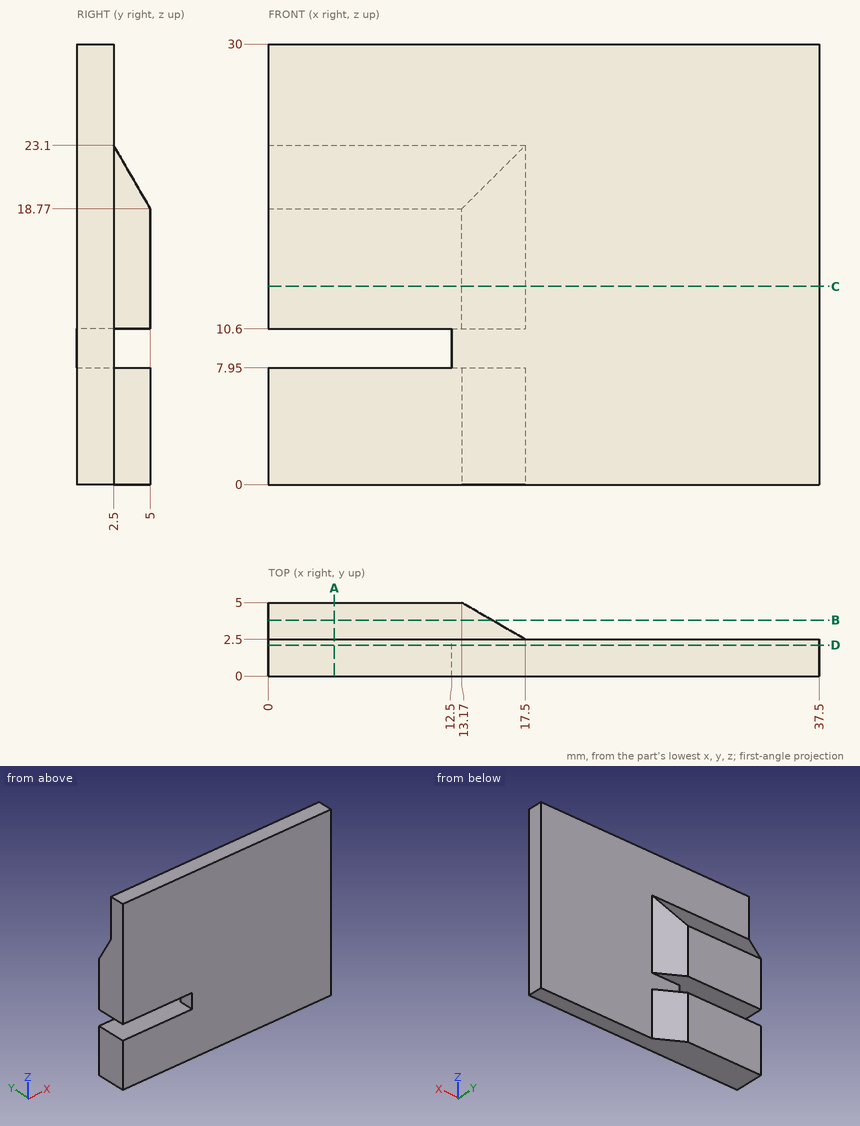
Here's the drawing with two shaded views (mm, measured from the low corner). I have some questions. Coordinates: 2 decimals unless noted, no trailing zeros. Write each loop counter-clockwise with the first axis right and the second up, starting at its lowest first coordinate (ties: lowest second). Pieces come first, ordered by that corner, then holes. Notation, with made-up numbers: M 38.5,-20.75 L 68.5,-20.75 A19 cw 68.5,13.25 Z; hole C 51,65 d4. An arc over 180 degrees is marked long. Use one line per item in the form item = value.
Q1. I need wall thicknesses on line 1 along Z through (x, y) = (4.5, 0.5); line 2 along Y through (x, z) = (23.5, 6.5); line 3 along X through (y, z) = (3.45, 16.75) (1 decimal). Which ranges of each line are inside material? Lowest first, please. Write a range as from..to.
Model answer:
line_1 = 0..7.95, 10.6..30
line_2 = 0..2.5
line_3 = 0..15.9
Q2. If we section it at A-A (x = 4.5): Write out the boundary of the cut face in (y, z).
Model answer:
outline = M 0,0 L 5,0 L 5,7.95 L 0,7.95 Z; M 0,10.6 L 5,10.6 L 5,18.77 L 2.5,23.1 L 2.5,30 L 0,30 Z
Q3. If we section it at B-B (y = 3.8): Write out the boundary of the cut face in (x, z), then the cut area to 4 significant figures.
Model answer:
outline = M 0,0 L 15.25,0 L 15.25,7.95 L 0,7.95 Z; M 0,10.6 L 15.25,10.6 L 15.25,20.85 L 0,20.85 Z
area = 277.5 mm^2
Q4. If we section it at D-D (y = 2.1): Write out the boundary of the cut face in (x, z), then the cut area to 3 significant figures.
Model answer:
outline = M 0,0 L 37.5,0 L 37.5,30 L 0,30 L 0,10.6 L 12.5,10.6 L 12.5,7.95 L 0,7.95 Z
area = 1,090 mm^2
Q5. For P1, Ø1.5, axis at x = 19.5, z = 4.5, coming from the +Y side, with a flat end and sliding along its axis, tell me the tip position at first contact or that it passes through.
Model answer:
P1 = 2.5
Q6. If we section it at C-C (z = 13.5): Write out the boundary of the cut face in (x, y).
Model answer:
outline = M 0,0 L 37.5,0 L 37.5,2.5 L 17.5,2.5 L 13.17,5 L 0,5 Z
